Autodesk Inventor part; units mm, degrees
ref_plane "YZ Plane" through (0, 0, 0) normal (1, 0, 0) x (0, 1, 0)
ref_plane "XZ Plane" through (0, 0, 0) normal (0, 1, 0) x (-1, 0, 0)
ref_plane "XY Plane" through (0, 0, 0) normal (0, 0, 1) x (1, 0, 0)
sketch "Náčrt1" plane through (0, 0, 0) normal (1, 0, 0) x (0, 1, 0)
  line L0 (0, 0) -> (37, 0)
  line L1 (37, 0) -> (37, -37)
  line L2 (37, -37) -> (0, -37)
  line L3 (0, -37) -> (0, 0)
  circle A0 centre (34, -34) radius 1.25
  circle A1 centre (3, -34) radius 1.25
  dimension "d0" = 37
  dimension "d1" = 37
  dimension "d2" = 2.5
  dimension "d3" = 3
  dimension "d4" = 3
  dimension "d5" = 3
extrude "Vysunutí1" add sketch "Náčrt1" along normal blind 3.5
sketch "Náčrt2" plane through (3.5, 0, 0) normal (1, 0, 0) x (0, 0, -1)
  line L0 (1, 27.25) -> (3.5, 27.25)
  line L1 (3.5, 27.25) -> (3.5, 9.75)
  line L2 (3.5, 9.75) -> (1, 9.75)
  line L3 (1, 9.75) -> (1, 27.25)
  line L4 (0, 37) -> (37, 37)
  line L5 (0, 37) -> (0, 0)
  dimension "d8" = 2.5
  dimension "d9" = 17.5
  dimension "d10" = 9.75
  dimension "d11" = 1
extrude "Vysunutí2" add sketch "Náčrt2" along normal blind 2.5
equation "\"d1\" = d0"
equation "\"d4\" = d3"
equation "\"d5\" = d4"
equation "\"d10\" = -0.5 * d9 + 0.5 * d0"
properties part number "SIM808 Module GSM GPRS GPS Breakout Board SIM808 for Arduino Raspberry"
Build history of the part. All positions in model axes, mm. A direction names the side the tool comes from. Round coordinates to 2 decimals unless told otherwise and drop trailing zeros. Loops run counter-clockwise (first coordinate to the right, second up) from the corner with the lowest first, then second, coordinate; pieces in that order, holes last. Notation, with made-up numbers: (-15, 42.5) -> (-10, 42.5) arc R26 ccw to (-10, 56.5) -> close; hole circle Ø9 at (-33.5, -1). An arc over 180 degrees is marked (long way). Answer in a Markdown table with one row per item.
Item 1: Saw through at D-D (x = 4.5). Write the cut outline in (y, z).
Answers below:
| item | result |
|---|---|
| outline | (9.75, -3.5) -> (27.25, -3.5) -> (27.25, -1) -> (9.75, -1) -> close |
Item 2: Saw through at B-B (y = 3). Write the cut outline in (x, z).
Answers below:
| item | result |
|---|---|
| outline | (0, -37) -> (3.5, -37) -> (3.5, -35.25) -> (0, -35.25) -> close; (0, -32.75) -> (3.5, -32.75) -> (3.5, 0) -> (0, 0) -> close |
Item 3: Which spindle directions (+Z, -Z, +X, -X, +Y, -Y) get a long thin tool onto all of the face, cutting with end or side? Do faces 1 (the flat face through (5, 19, -3.5)), 2 (the flat face through (5, 18, -1)), 3 (the flat face through (5, 9.75, -2)), 4 (the flat face through (5, 27.25, -2)). Say none if no direction does.
Answers below:
| item | result |
|---|---|
| face 1 | -Z, +X, +Y, -Y |
| face 2 | +Z, +X, +Y, -Y |
| face 3 | +Z, -Z, +X, -Y |
| face 4 | +Z, -Z, +X, +Y |
Item 4: Saw through at A-A (z = -34). Write the cut outline in (x, y), and give its area (3 significant figures).
Answers below:
| item | result |
|---|---|
| outline | (0, 0) -> (3.5, 0) -> (3.5, 1.75) -> (0, 1.75) -> close; (0, 4.25) -> (3.5, 4.25) -> (3.5, 32.75) -> (0, 32.75) -> close; (0, 35.25) -> (3.5, 35.25) -> (3.5, 37) -> (0, 37) -> close |
| area | 112 mm² |
Item 5: Mould opens along Y. For faces 5 (the flat face through (2, 0, -19)), 6 (the cylindrical face through (1.726, 34.577, -32.891)), 7 (the flat face through (6, 19, -2)) say: +Y half, -Y half, draft (parallel to the pull), parting line (faces both ways), or undercut.
Answers below:
| item | result |
|---|---|
| face 5 | -Y half |
| face 6 | undercut |
| face 7 | draft |
Item 6: Drill centre lines: L1, parallel to Z at x = 2.15, y = 34; L2, parallel to X at y = 14.5, z = -8; L3, parallel to Z at x = 1.3, y = 2. Where is each one in solid material? Low to high. Write a range as [from, to].
Answers below:
| item | result |
|---|---|
| L1 | z = [-37, -35.25], [-32.75, 0] |
| L2 | x = [0, 3.5] |
| L3 | z = [-37, -34.75], [-33.25, 0] |
Item 7: Saw through at C-C (y = 14.5). Write the cut outline in (x, z).
Answers below:
| item | result |
|---|---|
| outline | (0, -37) -> (3.5, -37) -> (3.5, -3.5) -> (6, -3.5) -> (6, -1) -> (3.5, -1) -> (3.5, 0) -> (0, 0) -> close |
Item 8: Pin check, flat tips, straight feed: pin 1 (12 mm diameter, centred on y = 9.5, z = -22, fed in from -X); pin 2 (1.2 mm diameter, centred on x = 5.5, z = -2, fed in from -Y); pin 3 (2 mm diameter, centred on x = 5, y = 27, fed in from -Z); pin 4 (1.2 mm diameter, centred on x = 4.5, z = -2.5, fed in from +Y). Stop position of each tip, or through.
Answers below:
| item | result |
|---|---|
| pin 1 | stops at x = 0 |
| pin 2 | stops at y = 9.75 |
| pin 3 | stops at z = -3.5 |
| pin 4 | stops at y = 27.25 |
